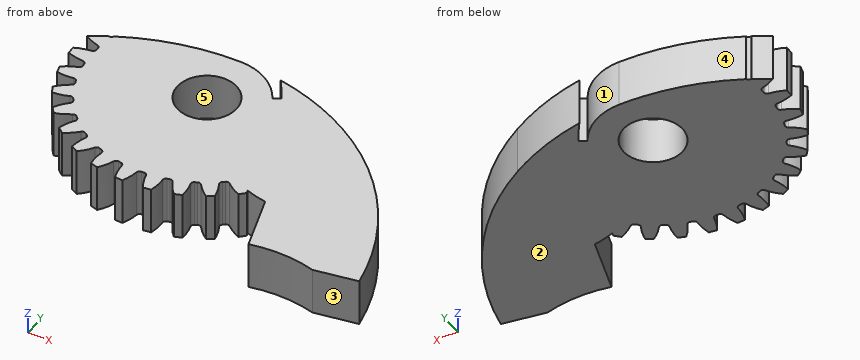
from build123d import *

# Parameters (mm, degrees)
SKETCH3_R               = 40.64
GEARBODY_DEPTH          = 9.652
TOOTHCUT_DEPTH          = 59.278472046
CIRPATTERN1_COUNT       = 30
SCALE1_SCALE_X          = 0.666666667
SCALE1_SCALE_Y          = 0.666666667
SCALE1_SCALE_Z          = 1
BOREDIA_R               = 6.025500014
BORE_DEPTH              = 12700
CUT_EXTRUDE1_DEPTH      = 40.49986663
BOSS_EXTRUDE1_DEPTH     = 9.652
BODY_TUBE_CUT_OUT_DEPTH = 59.606597669


with BuildPart() as part:
    # Sketch3 → gearBody (new body)
    with BuildSketch(Plane.XY):
        Circle(SKETCH3_R)
    extrude(amount=GEARBODY_DEPTH)

    # Sketch2 → toothCut (cut, through all)
    with BuildSketch(Plane.XY):
        with BuildLine():
            ThreePointArc((34.901466352, -2.640387833), (34.929801576, -2.234493965), (34.953416534, -1.828298136))
            ThreePointArc((34.953416534, -1.828298136), (35.218972856, -1.205360668), (35.823821616, -0.900845929))
            ThreePointArc((35.823821616, -0.900845929), (41.902420255, 1.180053047), (46.567899911, 5.597382731))
            ThreePointArc((46.567899911, 5.597382731), (46.807414621, -2.994316622), (45.4750933, -11.485464069))
            ThreePointArc((45.4750933, -11.485464069), (41.410501506, -6.509663078), (35.646600115, -3.671187658))
            ThreePointArc((35.646600115, -3.671187658), (35.08548304, -3.292084932), (34.901466352, -2.640387833))
        make_face()
    toothcut = extrude(amount=TOOTHCUT_DEPTH, mode=Mode.SUBTRACT)

    # CirPattern1: toothCut ×30 about axis
    cirpattern1_axis = Axis((0, 0, 0), (0, 0, 1))
    for i in range(1, CIRPATTERN1_COUNT):
        add(toothcut.rotate(cirpattern1_axis, i * 360 / CIRPATTERN1_COUNT), mode=Mode.SUBTRACT)


with BuildPart() as part_1:
    # Scale1: scaled about (0, 0, 4.826)
    add(part.part.scale((SCALE1_SCALE_X, SCALE1_SCALE_Y, SCALE1_SCALE_Z), about=(0, 0, 4.826)))

    # boreDia → bore (cut, symmetric)
    with BuildSketch(Plane.XY):
        Circle(BOREDIA_R)
    extrude(amount=BORE_DEPTH, both=True, mode=Mode.SUBTRACT)

    # Sketch4 → Cut-Extrude1 (cut, through all)
    with BuildSketch(Plane.XY.offset(9.652)):
        with BuildLine():
            ThreePointArc((-27.126729009, 3.341060233), (0, 11.43), (27.126729009, 3.341060233))
            ThreePointArc((27.126729009, 3.341060233), (0, 27.33170522), (-27.126729009, 3.341060233))
        make_face()
    extrude(amount=-CUT_EXTRUDE1_DEPTH, mode=Mode.SUBTRACT)

    # Sketch5 → Boss-Extrude1 (add)
    with BuildSketch(Plane.XY.offset(9.652)):
        with BuildLine():
            Line((23.424769806, -19.215611802), (26.959165805, -30.742024145))
            ThreePointArc((26.959165805, -30.742024145), (33.569316663, -30.066976699), (40.144948283, -31.021362479))
            Line((40.144948283, -31.021362479), (48.777528007, -29.49920576))
            ThreePointArc((48.777528007, -29.49920576), (34.808245264, -2.863556342), (8.00379846, 10.779035488))
            add(Edge.make_bspline(
                [(8.00379846, 10.779035488), (4.700723166, -16.48766374), (23.424769806, -19.215611802)],
                knots=[0, 0, 0, 1, 1, 1], degree=2))
        make_face()
    extrude(amount=-BOSS_EXTRUDE1_DEPTH)

    # Sketch6 → Body Tube Cut Out (cut, through all)
    with BuildSketch(Plane.XY.offset(9.652)):
        with BuildLine():
            Line((11.262487171, 6.5024), (9.898670365, 5.715))
            ThreePointArc((9.898670365, 5.715), (5.715, 9.898670365), (0, 11.43))
            ThreePointArc((0, 11.43), (4.300943022, 11.242910221), (8.569394121, 10.683054275))
            ThreePointArc((8.569394121, 10.683054275), (9.966823016, 8.625504533), (11.262487171, 6.5024))
        make_face()
    extrude(amount=-BODY_TUBE_CUT_OUT_DEPTH, mode=Mode.SUBTRACT)


solid = part_1.part
Geometry check sheet. Reference: the model listing, model coordinates, mm. Face numbers are marked on the shaded views. A direction names the side the tool comes from. Give positions to 0.01 mm unless a question says otherwise; leave off trailing zeros. Use one line per item in the form item = value.
1) Depth check by flat-ended pin: pin 1 Ø1 at (y, z) = (-6.5, 4.5) entering from -X; pin 2 Ø9.5 at (x, y) = (0, 0) entering from +Z; pin 3 Ø2 at (y, z) = (-18, 1.5) entering from +X; pin 4 Ø1 at (y, z) = (-7.5, 6.5) entering from +X. Enter the tip coordinate at first touch or a pass-through.
Working result:
pin_1 = -26.42
pin_2 = through
pin_3 = 45.7
pin_4 = 39.33
2) Draft check along X on the marked faces 3, 4 and 5. Enter one of: released by +X, released by -X, zero draft, split by the parting line, or undercut.
Working result:
face_3 = released by +X
face_4 = released by -X
face_5 = undercut
3) Material ranges on probe 1 along Y at (x, z) = (0.5, 1.75); probe 2 along X at (y, z) = (-4, 1); probe 3 along X at (y, z) = (-17, 5.25), recorded low to high. Write a range as from..to.
Working result:
probe_1 = -23.36..-6, 6..11.42
probe_2 = -23.09..-4.51, 4.51..35.92
probe_3 = -21.1..-19.55, -16.31..44.81
4) Access from +Z, -Z, +X, -X, +Y, -Y to the whole of each face (thin tool, end or side, straight path). Record for the marked faces 1 and 2.
Working result:
face_1 = +Z, -Z
face_2 = -Z, +X, -X, +Y, -Y
